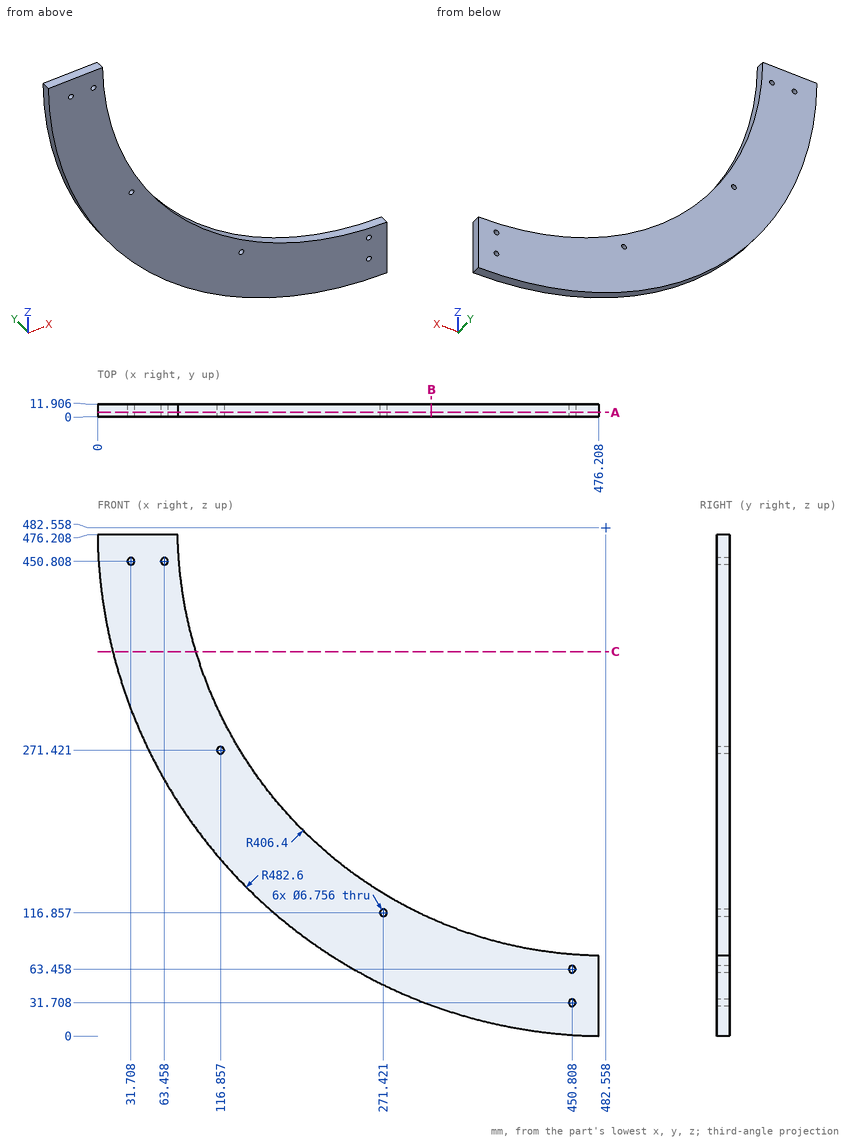
Check sheet for the drawn part. Datum: minimum x, y, z corner. Units: mm. Round coordinates to 2 decimals unless told otherwise and drop trailing zeros. Write each loop counter-clockwise with the first axis right and the second up, starting at its lowest first coordinate (ties: lowest second). Pieces come first, ordered by that corner, then holes. Notation, with made-up numbers: (-32.75, 2) -> (-17.75, 2) arc R26 cw to (-17.75, 26) -> close; hole circle Ø2 at (50, 45.5). An arc over 180 degrees is marked (long way). Put each result on its own line as item: value.
(1) Sectioned sample at A-A (y = 4). Enter the section's corners in (x, z), plus the area to 3 significant figures.
Values found:
outline: (0, 476.21) arc R482.6 ccw to (476.21, 0) -> (476.21, 76.21) arc R406.4 cw to (76.21, 476.21) -> close; hole circle Ø6.76 at (31.71, 450.81); hole circle Ø6.76 at (63.46, 450.81); hole circle Ø6.76 at (116.86, 271.42); hole circle Ø6.76 at (271.42, 116.86); hole circle Ø6.76 at (450.81, 31.71); hole circle Ø6.76 at (450.81, 63.46)
area: 52,000 mm^2
(2) Material ranges on line 1 (X direction, y = 9, z = 64) (1 decimal); line 2 (Z direction, x = 313, y = 2.5) (1 decimal); line 3 (Z direction, x = 300, y = 7.75), recorded low to high.
Values found:
line 1: x = 242.3 to 447.5, 454.1 to 476.2
line 2: z = 30.7 to 113.2
line 3: z = 35.82 to 119.47
(3) Sectioned sample at B-B (x = 317). Enter the section's corners in (y, z) (1 decimal), plus the area to 3 significant figures.
Values found:
outline: (0, 29.2) -> (11.9, 29.2) -> (11.9, 111.4) -> (0, 111.4) -> close
area: 978 mm^2
(4) Go/stop test with flat-tipped pins: pin 1 Ø3 at (y, z) = (4.5, 246.5) entering from -X; pin 2 Ø5 at (x, y) = (228.5, 2) entering from -Z; pin 3 Ø5 at (y, z) = (8, 352.5) entering from -X. Record where each tip stops, or that it passes through.
Values found:
pin 1: stops at x = 60.79
pin 2: stops at z = 70.71
pin 3: stops at x = 17.12
(5) Sectioned sample at C-C (z = 365). Enter the section's corners in (x, y) (1 decimal).
Values found:
outline: (14.5, 0) -> (93.5, 0) -> (93.5, 11.9) -> (14.5, 11.9) -> close
